For this review, use the dimensioned drawing (mm, ordinates from the lowest corner) and the shaded views. A direction names the side the tool comes from. Round coordinates to 2 decimals unless told otherwise and drop trailing zeros. Write each loop counter-clockwise with the first axis right and the second up, starting at its lowest first coordinate (ties: lowest second). Pieces come first, ordered by that corner, then holes.
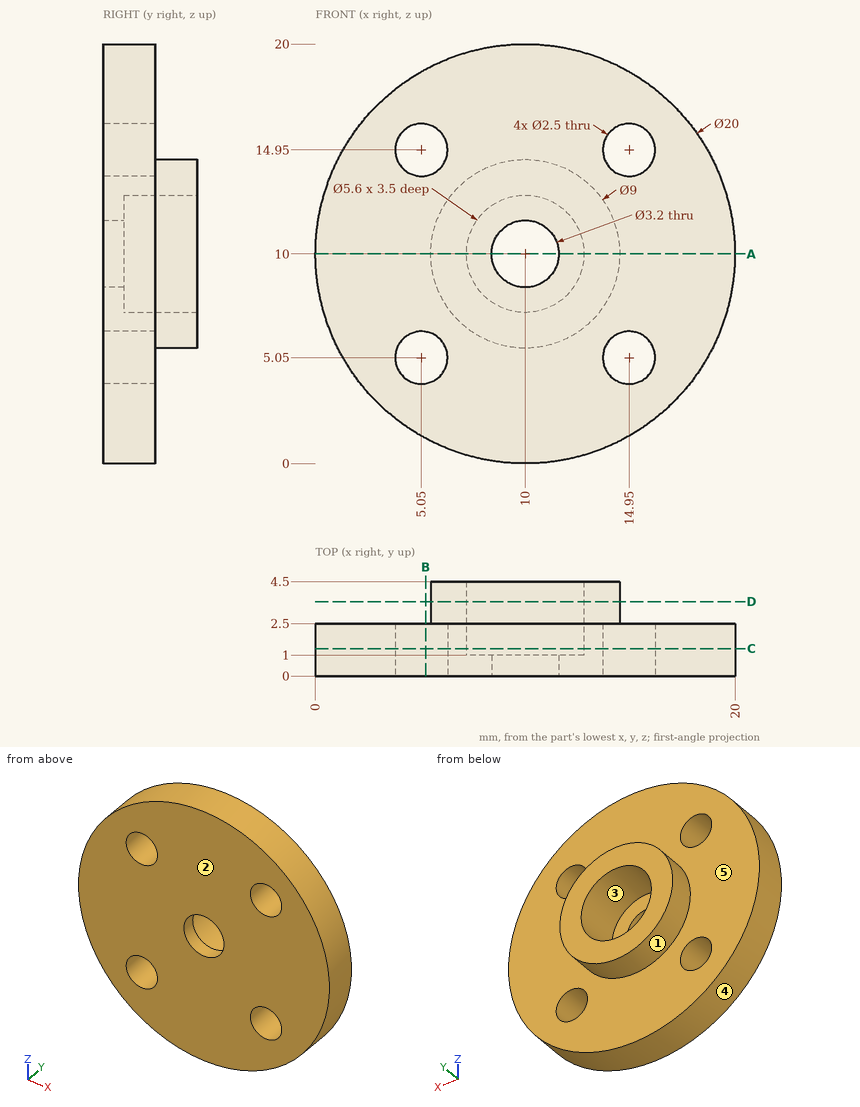
(1) We need section A-A, the plane z = 10. Give the boundary of the cut face in (x, y).
Geometry check:
outline: (0, 0) - (8.4, 0) - (8.4, 1) - (7.2, 1) - (7.2, 4.5) - (5.5, 4.5) - (5.5, 2.5) - (0, 2.5) - close; (11.6, 0) - (20, 0) - (20, 2.5) - (14.5, 2.5) - (14.5, 4.5) - (12.8, 4.5) - (12.8, 1) - (11.6, 1) - close
(2) For the marked faces 1 and 2, list the 3-axis set-ups (+Z, -Z, +X, -X, +Y, -Y) from which the entire face can be reached by the end or side of a thin tool; tool diameter is ignored.
Geometry check:
face 1: +Y
face 2: +Z, -Z, +X, -X, -Y
(3) For line 1 along X through (y, z) = (0.3, 10); line 2 along Z through (x, y) = (5.5, 1.6); line 3 along X through (y, z) = (1.95, 14.75) (1 decimal), list the stretches that pass through material, from the lowest coordinate up.
Geometry check:
line 1: x = 0 to 8.4, 11.6 to 20
line 2: z = 1.07 to 3.88, 6.22 to 13.78, 16.12 to 18.93
line 3: x = 1.2 to 3.8, 6.3 to 13.7, 16.2 to 18.8
(4) We need section C-C, the plane y = 1.3. Give the boundary of the cut face in (x, z), and give its area (3 significant figures).
Geometry check:
outline: circle Ø20 at (10, 10); hole circle Ø2.5 at (5.05, 5.05); hole circle Ø2.5 at (5.05, 14.95); hole circle Ø5.6 at (10, 10); hole circle Ø2.5 at (14.95, 5.05); hole circle Ø2.5 at (14.95, 14.95)
area: 270 mm2
(5) For pin 1 Ø1.5 at (x, z) = (14.95, 5.05) entering from +Y; pin 2 Ø3 at (x, z) = (14.95, 14.95) entering from +Y, all flat-tipped, find the tip position at first contact; note any pin that passes through.
Geometry check:
pin 1: passes through
pin 2: stops at y = 2.5
(6) We need section D-D, the plane y = 3.55. Give the boundary of the cut face in (x, z), and give its area (3 significant figures).
Geometry check:
outline: circle Ø9 at (10, 10); hole circle Ø5.6 at (10, 10)
area: 39.0 mm2
(7) Mouldability with a two-part tool opening along X and no side actions: class the marked faces 3, 4 and 5 as pulls with the +X half, pulls with the -X half, needs draft (parallel to the pull), parting line crosses it, or undercut.
Geometry check:
face 3: undercut
face 4: parting line crosses it
face 5: needs draft
(8) We need section B-B, the plane x = 5.25. Give the boundary of the cut face in (y, z).
Geometry check:
outline: (0, 1.2) - (2.5, 1.2) - (2.5, 3.82) - (0, 3.82) - close; (0, 6.28) - (2.5, 6.28) - (2.5, 13.72) - (0, 13.72) - close; (0, 16.18) - (2.5, 16.18) - (2.5, 18.8) - (0, 18.8) - close
